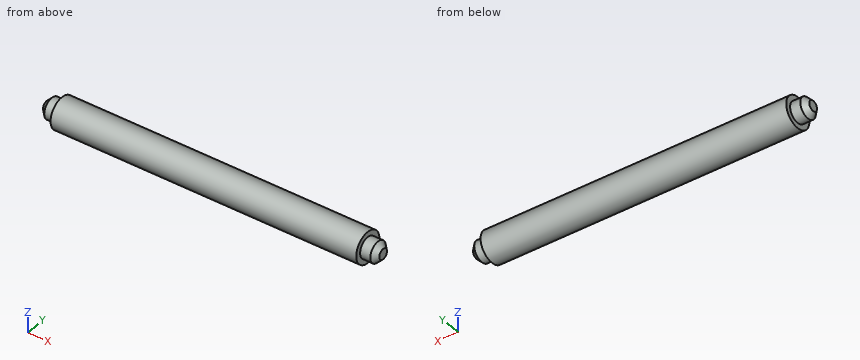
from build123d import *

# Parameters (mm, degrees)
CHANFREIN1_SIZE = 1


with BuildPart() as part:
    # Esquisse1 → Base-Révolution (revolve)
    with BuildSketch(Plane.XY, mode=Mode.PRIVATE) as base_r_volution_sk:
        Polygon((-33, 2), (-33, 0), (33, 0), (33, 2), (30, 2), (30, 3), (-30, 3), (-30, 2), align=None)
    revolve(base_r_volution_sk.sketch.rotate(Axis((-77, 0, 0), (1, 0, 0)), 90), axis=Axis((-77, 0, 0), (1, 0, 0)))

    # Chanfrein1
    chanfrein1_edges = [part.edges().sort_by_distance(p)[0] for p in [
        (-33, 0, -2),
        (33, 0, -2),
    ]]
    chamfer(chanfrein1_edges, length=CHANFREIN1_SIZE)


solid = part.part
Here's how the part is built. I have some questions about the finished solid (model axes, mm). Give positions to 0.01 mm unless a question says otherwise; leave off trailing zeros. Loops run counter-clockwise (first coordinate to the right, second up) from the corner with the lowest first, then second, coordinate; pieces in that order, holes last. Notation, with made-up numbers: (-13, 33) -> (46, 33) arc R18 cw to (46, 53) -> close; hole circle Ø5 at (21, 57). An arc over 180 degrees is marked (long way). Answer as a JSON object with one key per item and string values. Group by question number.
Item 1: Will these pins go through, and if not, where does the flat tip stop? pin 1 (1 mm diameter, centred on x = -18, z = -2, fed in from -Y); pin 2 (1 mm diameter, centred on x = 10.5, y = -1, fed in from +Z); pin 3 (1.5 mm diameter, centred on x = -5, z = -2, fed in from -Y); pin 4 (1.5 mm diameter, centred on y = 1.5, z = -0.5, fed in from -X).
Item 2: I need wall thicknesses on L1, parallel to X at y = -0.15, z = -1; L2, parallel to X at y = 2.2, z = -2; L3, parallel to Z at x = -28, y = 0.85. Which ranges of each line are inside material? Lowest first, please.
Item 3: Imagine slicing it at C-C on x = 0. Write out the boundary of the cut face in (y, z), then the cut area to 3 significant figures.
Item 4: Imagine slicing it at A-A on y = 0. Write out the boundary of the cut face in (x, z).
Answer list:
{
 "1": {"pin 1": "stops at y = -2.6", "pin 2": "stops at z = 2.96", "pin 3": "stops at y = -2.73", "pin 4": "stops at x = -33"},
 "2": {"L1": "x = -32.99 to 32.99", "L2": "x = -30 to 30", "L3": "z = -2.88 to 2.88"},
 "3": {"outline": "circle Ø6 at (0, 0)", "area": "28.3 mm2"},
 "4": {"outline": "(-33, -1) -> (-32, -2) -> (-30, -2) -> (-30, -3) -> (30, -3) -> (30, -2) -> (32, -2) -> (33, -1) -> (33, 1) -> (32, 2) -> (30, 2) -> (30, 3) -> (-30, 3) -> (-30, 2) -> (-32, 2) -> (-33, 1) -> close"}
}
